Work out the finished part from the listing and answer in its coordinate system (mm). Round coordinates to 2 decimals unless told otherwise and drop trailing zeros. Order: outer loops, then holes, each group sorted by start corner. A loop starts at its lowest first (then second) coordinate and runs counter-clockwise, first axis right, second up. Notation, with made-up numbers: (3.5, 44) - (35.5, 44) arc R13 cw to (35.5, 54) - close; hole circle Ø10 at (17, -9). An arc over 180 degrees is marked (long way). Use CSV: the item, a comma, the result in double quotes.
Autodesk Inventor part; units mm, degrees
ref_plane "YZ Plane" through (0, 0, 0) normal (1, 0, 0) x (0, 1, 0)
ref_plane "XZ Plane" through (0, 0, 0) normal (0, 1, 0) x (-1, 0, 0)
ref_plane "XY Plane" through (0, 0, 0) normal (0, 0, 1) x (1, 0, 0)
sketch "Sketch1" plane through (0, 0, 0) normal (0, 0, 1) x (1, 0, 0)
  circle A0 centre (0, 0) radius 4.5
  circle A1 centre (0, 0) radius 2.5
  dimension "d0" = 9
  dimension "d1" = 5
extrude "Extrusion1" add sketch "Sketch1" along normal blind 11
sketch "Sketch2" plane through (0, 0, 0) normal (1, 0, 0) x (0, 1, 0)
  circle A0 centre (5.15, 7.65) radius 1.65
  line L0 (-4.5, 0) -> (4.5, 0)
  line L1 (0, 0) -> (0, 16.0894)
  dimension "d7" = 7.65
  dimension "d8" = 5.15
  dimension "d9" = 3.3
revolve "Revolution1" cut sketch "Sketch2" angle 360 about axis through (0, 0, 0) along (0, 0, 1)
sketch "Sketch3" plane through (0, 0, 0) normal (1, 0, 0) x (0, 1, 0)
  circle A0 centre (0, 3.1) radius 1.25
  point P0 (0, 0)
  dimension "d11" = 2.5
  dimension "d12" = 3.1
extrude "Extrusion2" cut sketch "Sketch3" against normal blind 11
thread "Thread1"
properties part number "MK8_Drive_Gear"
(1) Find section C-C (z = 1.25). Determine the outline of the cut face in (x, y).
Findings below:
outline,"circle Ø9 at (0, 0); hole circle Ø5 at (0, 0)"
(2) Find the intervals of material crossed by L1, parallel to Y at x = 0, z = 5; L2, parallel to Y at x = 0.5, z = 4, in increasing order. Write a range as from..to.
Findings below:
L1,"y = -4.5..-2.5, 2.5..4.5"
L2,"y = -4.47..-2.45, 2.45..4.47"
(3) Each of these flat-tipped pins is pushed along its axis until it touches: pin 1 (2 mm diameter, centred on x = -1, y = 1, fed in from -Z); pin 2 (1.5 mm diameter, centred on y = -1, z = 9.5, fed in from +X); pin 3 (3 mm diameter, centred on x = 2, z = 2.5, fed in from +Y); pin 4 (1 mm diameter, centred on y = -1, z = 8, fed in from -X). Where does it stop, or does it pass through?
Findings below:
pin 1,"passes through"
pin 2,"stops at x = 4.49"
pin 3,"stops at y = 4.47"
pin 4,"stops at x = -3.62"
(4) Find section B-B (y = 0). Determine the outline of the cut face in (x, z).
Findings below:
outline,"(-4.5, 0) - (-2.5, 0) - (-2.5, 1.85) - (-4.5, 1.85) - close; (-4.5, 4.35) - (-2.5, 4.35) - (-2.5, 11) - (-4.5, 11) - (-4.5, 9.17) arc R1.65 cw to (-4.5, 6.13) - close; (2.5, 0) - (4.5, 0) - (4.5, 6.13) arc R1.65 cw to (4.5, 9.17) - (4.5, 11) - (2.5, 11) - close"
(5) Find section D-D (z = 3.75). Determine the outline of the cut face in (x, y), and give its area (3 significant figures).
Findings below:
outline,"(-4.37, -1.07) arc R4.5 ccw (long way) to (-4.37, 1.07) - (-2.26, 1.07) arc R2.5 cw (long way) to (-2.26, -1.07) - close"
area,"39.6 mm²"
(6) The mould has two halves that part along Y. Classify faces 1 (the flat face through (2, -2, 11)), 2 (the cylindrical face through (-3.32, -0.27, 1.88)), 3 (the cylindrical face through (-0.59, -4.46, 10.07)): released by +Y, released by -Y, zero draft, split by the parting line, or undercut.
Findings below:
face 1,"zero draft"
face 2,"undercut"
face 3,"split by the parting line"
(7) Find section A-A (x = 0). Determine the outline of the cut face in (y, z), and give its area (3 significant figures).
Findings below:
outline,"(-4.5, 0) - (-2.5, 0) - (-2.5, 11) - (-4.5, 11) - (-4.5, 9.17) arc R1.65 cw to (-4.5, 6.13) - close; (2.5, 0) - (4.5, 0) - (4.5, 6.13) arc R1.65 cw to (4.5, 9.17) - (4.5, 11) - (2.5, 11) - close"
area,"39.6 mm²"
